Geometry check sheet. Reference: the model listing, model coordinates, mm. Face numbers are marked on the shaded views. A direction names the side the tool comes from. Give positions to 0.01 mm unless a question says otherwise; leave off trailing zeros. Loops run counter-clockwise (first coordinate to the right, second up) from the corner with the lowest first, then second, coordinate; pieces in that order, holes last. Notation, with made-up numbers: (-23.75, -12.75) - (-11.75, -12.75) arc R25 cw to (-11.75, 24.25) - close; hole circle Ø1 at (-39, -4.75). An arc over 180 degrees is marked (long way). Use a Markdown table: item, result. Add a question column.
1. Cross-section at B-B on y = 0. Enter the section's corners in (x, z), and give its area (3 significant figures).
2. Cross-section at C-C on x = 0. Count the separate pieces of the cut face and the enclosed holes in it, and give its area (3 significant figures).
3. Cross-section at A-A on z = 0. Enter the section's corners in (x, y).
4. Cross-section at D-D on y = 7.5. Enter the section's corners in (x, z).
5. Material ranges on L1, parallel to Z at x = 1.45, y = -5; L2, parallel to X at y = -7.5, z = 1.8; L3, parallel to Y at x = 0, z = 1.95, recorded low to high.
6. Set-up check for the marked faces 1 and 2: record each of +Z, -Z, +X, -X, +Y, -Y from which the full face is reachable in a straight line by a thin tool's end or side.
7. Draft check along Y on the marked faces 3, 4 and 5. Enter one of: pulls with the +Y half, pulls with the -Y half, needs draft (parallel to the pull), parting line crosses it, or undercut.
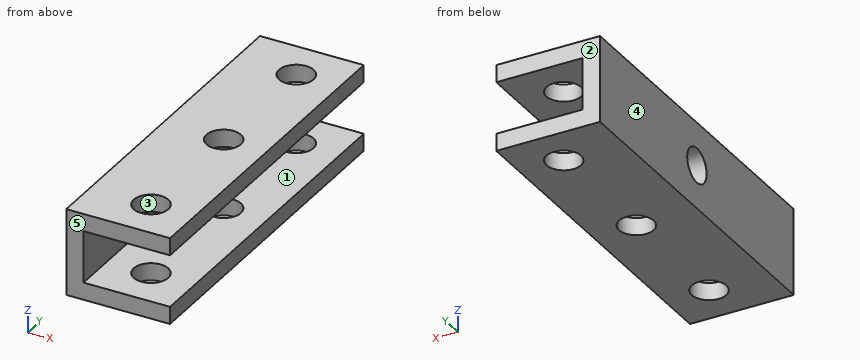
from build123d import *

# Parameters (mm, degrees)
F1_DEPTH = 10
F2_R     = 1
F3_DEPTH = 2.5
F4_R     = 1
F5_DEPTH = 5


with BuildPart() as f1:
    # F0 (on Front) → F1 (new body, symmetric)
    with BuildSketch(Plane.XZ):
        Polygon((-2.5, 1.5), (2.5, 1.5), (2.5, 2.5), (-3.5, 2.5), (-3.5, -2.5), (2.5, -2.5), (2.5, -1.5), (-2.5, -1.5), align=None)
    extrude(amount=F1_DEPTH, both=True)

    # F2 (on Top) → F3 (cut, symmetric)
    with BuildSketch(Plane.XY):
        with Locations((0, 7.5)):
            Circle(F2_R)
        with Locations((0, -7.5)):
            Circle(F2_R)
        Circle(F2_R)
    extrude(amount=F3_DEPTH, both=True, mode=Mode.SUBTRACT)

    # F4 (on Right) → F5 (cut, symmetric)
    with BuildSketch(Plane.YZ):
        Circle(F4_R)
    extrude(amount=F5_DEPTH, both=True, mode=Mode.SUBTRACT)


solid = f1.part
Values found:
| question | item | result |
|---|---|---|
| 1 | outline | (-3.5, -2.5) - (-1, -2.5) - (-1, -1.5) - (-2.5, -1.5) - (-2.5, -1) - (-3.5, -1) - close; (-3.5, 1) - (-2.5, 1) - (-2.5, 1.5) - (-1, 1.5) - (-1, 2.5) - (-3.5, 2.5) - close; (1, -2.5) - (2.5, -2.5) - (2.5, -1.5) - (1, -1.5) - close; (1, 1.5) - (2.5, 1.5) - (2.5, 2.5) - (1, 2.5) - close |
| 1 | area | 9.00 mm2 |
| 2 | separate pieces | 8 |
| 2 | enclosed holes | 0 |
| 2 | area | 28.0 mm2 |
| 3 | outline | (-3.5, -10) - (-2.5, -10) - (-2.5, -1) - (-3.5, -1) - close; (-3.5, 1) - (-2.5, 1) - (-2.5, 10) - (-3.5, 10) - close |
| 4 | outline | (-3.5, -2.5) - (-1, -2.5) - (-1, -1.5) - (-2.5, -1.5) - (-2.5, 1.5) - (-1, 1.5) - (-1, 2.5) - (-3.5, 2.5) - close; (1, -2.5) - (2.5, -2.5) - (2.5, -1.5) - (1, -1.5) - close; (1, 1.5) - (2.5, 1.5) - (2.5, 2.5) - (1, 2.5) - close |
| 5 | L1 | z = -2.5 to -1.5, 1.5 to 2.5 |
| 5 | L2 | x = -3.5 to -1, 1 to 2.5 |
| 5 | L3 | y = -10 to -8.5, -6.5 to -1, 1 to 6.5, 8.5 to 10 |
| 6 | face 1 | +X, +Y, -Y |
| 6 | face 2 | +Z, -Z, +X, -X, +Y |
| 7 | face 3 | undercut |
| 7 | face 4 | needs draft |
| 7 | face 5 | pulls with the -Y half |
